```python
from build123d import *

# Parameters (mm, degrees)
F3_R     = 9.5
F3_R_2   = 7.5
F3_R_3   = 4.9
F4_DEPTH = 1
F6_DEPTH = 9
F7_DEPTH = 15.5


with BuildPart() as f4:
    # F3 (on Top) → F4 (new body)
    with BuildSketch(Plane.XY):
        Circle(F3_R)
        Circle(F3_R_2, mode=Mode.SUBTRACT)
        Circle(F3_R_2)
        Circle(F3_R_3, mode=Mode.SUBTRACT)
        Circle(F3_R_3)
        with BuildLine():
            ThreePointArc((-2.2847319318, -2.45), (-3.35, 0), (-2.2847319318, 2.45))
            Line((-2.2847319318, 2.45), (2.2847319318, 2.45))
            ThreePointArc((2.2847319318, 2.45), (3.35, 0), (2.2847319318, -2.45))
            Line((2.2847319318, -2.45), (-2.2847319318, -2.45))
        make_face(mode=Mode.SUBTRACT)
    extrude(amount=F4_DEPTH)


with BuildPart() as f5_1:
    # F5: copy of F4
    add(f4.part.moved(Location((0, 0, 6))))


with BuildPart() as f6:
    # F3 (on Top) → F6 (new body)
    with BuildSketch(Plane.XY):
        Circle(F3_R_2)
        Circle(F3_R_3, mode=Mode.SUBTRACT)
        Circle(F3_R_3)
        with BuildLine():
            ThreePointArc((-2.2847319318, -2.45), (-3.35, 0), (-2.2847319318, 2.45))
            Line((-2.2847319318, 2.45), (2.2847319318, 2.45))
            ThreePointArc((2.2847319318, 2.45), (3.35, 0), (2.2847319318, -2.45))
            Line((2.2847319318, -2.45), (-2.2847319318, -2.45))
        make_face(mode=Mode.SUBTRACT)
    extrude(amount=F6_DEPTH)


with BuildPart() as f4_1:
    add(f4.part)

    add(f5_1.part)  # F7 merges F5_1

    add(f6.part)  # F7 merges F6
    # F3 (on Top) → F7 (join)
    with BuildSketch(Plane.XY):
        Circle(F3_R_3)
        with BuildLine():
            ThreePointArc((-2.2847319318, -2.45), (-3.35, 0), (-2.2847319318, 2.45))
            Line((-2.2847319318, 2.45), (2.2847319318, 2.45))
            ThreePointArc((2.2847319318, 2.45), (3.35, 0), (2.2847319318, -2.45))
            Line((2.2847319318, -2.45), (-2.2847319318, -2.45))
        make_face(mode=Mode.SUBTRACT)
    extrude(amount=F7_DEPTH)

    # F8 (on Front) → F9 (revolve)
    with BuildSketch(Plane.XZ):
        Polygon((5.15, 14.75), (4.9, 15.5), (4.9, 14), align=None)
    revolve(axis=Axis((0, 0, 8.7542282417), (0, 0, 1)))


solid = f4_1.part
```
Check sheet for the modelled part. Datum: model origin and axes. Units: mm. A direction names the side the tool comes from. Give positions to 0.01 mm unless a question says otherwise; leave off trailing zeros. Write each loop counter-clockwise with the first axis right and the second up, starting at its lowest first coordinate (ties: lowest second). Pieces come first, ordered by that corner, then holes.
Item 1: Cross-section at A-A (x = 0). Enter the section's corners in (y, z), and give its area (3 significant figures).
Item 2: Scan lines: L1, parallel to Y at x = 0, z = 6.75; L2, parallel to Z at x = -8.5, y = -1; L3, parallel to X at y = 0, z = 8.5. Record each from-to range of solid material in increasing order.
Item 3: Cross-section at B-B (y = 0). Enter the section's corners in (x, z).
Item 4: Access from +Z, -Z, +X, -X, +Y, -Y to the whole of each face (thin tool, end or side, straight path). Record for faces 1 (the face through (0, -3, 15.5)), 2 (the face through (0, 2.45, 8)), 3 (the face through (-1.062, -4.783, 11.465)), 4 (the face through (1, 8, 7)).
Item 5: Draft check along Z on faces 5 (the face through (1, 8, 1)), 6 (the face through (4, 0, 0)), 7 (the face through (0, -2.45, 8)). Enter one of: released by +Z, released by -Z, zero draft, split by the parting line, or undercut.
Item 6: Cross-section at C-C (z = 8.75). Enter the section's corners in (x, y).
Item 7: Gauge pin test, flat ends, axial feed: pin 1 (1 mm diameter, centred on y = 1, z = 13, fed in from +X); pin 2 (1.4 mm diameter, centred on x = 1, z = 4.5, fed in from -Y); pin 3 (5 mm diameter, centred on x = 6.5, z = 7, fed in from -Y). Record the tip position at first contact, or that the pin passes through.
Item 8: Cross-section at D-D (y = -5.5). Enter the section's corners in (x, z).
Report:
1. outline: (-9.5, 0) - (-2.45, 0) - (-2.45, 15.5) - (-4.9, 15.5) - (-5.15, 14.75) - (-4.9, 14) - (-4.9, 9) - (-7.5, 9) - (-7.5, 7) - (-9.5, 7) - (-9.5, 6) - (-7.5, 6) - (-7.5, 1) - (-9.5, 1) - close; (2.45, 0) - (9.5, 0) - (9.5, 1) - (7.5, 1) - (7.5, 6) - (9.5, 6) - (9.5, 7) - (7.5, 7) - (7.5, 9) - (4.9, 9) - (4.9, 14) - (5.15, 14.75) - (4.9, 15.5) - (2.45, 15.5) - close
1. area: 131 mm2
2. L1: y = -9.5 to -2.45, 2.45 to 9.5
2. L2: z = 0 to 1, 6 to 7
2. L3: x = -7.5 to -3.35, 3.35 to 7.5
3. outline: (-9.5, 0) - (-3.35, 0) - (-3.35, 15.5) - (-4.9, 15.5) - (-5.15, 14.75) - (-4.9, 14) - (-4.9, 9) - (-7.5, 9) - (-7.5, 7) - (-9.5, 7) - (-9.5, 6) - (-7.5, 6) - (-7.5, 1) - (-9.5, 1) - close; (3.35, 0) - (9.5, 0) - (9.5, 1) - (7.5, 1) - (7.5, 6) - (9.5, 6) - (9.5, 7) - (7.5, 7) - (7.5, 9) - (4.9, 9) - (4.9, 14) - (5.15, 14.75) - (4.9, 15.5) - (3.35, 15.5) - close
4. face 1: +Z, +X, -X, +Y, -Y
4. face 2: +Z, -Z
4. face 3: none
4. face 4: +Z
5. face 5: undercut
5. face 6: released by -Z
5. face 7: zero draft
6. outline: circle Ø15 at (0, 0); hole (-2.28, -2.45) - (2.28, -2.45) arc R3.35 ccw to (2.28, 2.45) - (-2.28, 2.45) arc R3.35 ccw to start
7. pin 1: stops at x = 4.87
7. pin 2: stops at y = -7.49
7. pin 3: stops at y = -8.62
8. outline: (-7.75, 0) - (7.75, 0) - (7.75, 1) - (5.1, 1) - (5.1, 6) - (7.75, 6) - (7.75, 7) - (5.1, 7) - (5.1, 9) - (-5.1, 9) - (-5.1, 7) - (-7.75, 7) - (-7.75, 6) - (-5.1, 6) - (-5.1, 1) - (-7.75, 1) - close
